CAD build for the part. Positions are in the model's coordinates, mm. Face numbers are marked on the shaded views. A direction names the side the tool comes from. Round coordinates to 2 decimals unless told otherwise and drop trailing zeros. Write each loop counter-clockwise with the first axis right and the second up, starting at its lowest first coordinate (ties: lowest second). Pieces come first, ordered by that corner, then holes. Notation, with made-up numbers: (6.25, -13) - (14.25, -13) arc R14 cw to (14.25, 6) - close; hole circle Ø10 at (-18.5, 67.5). An arc over 180 degrees is marked (long way). Answer in a Markdown table with one row per item.
```python
from build123d import *

# Parameters (mm, degrees)
BOSS_EXTRUDE1_DEPTH = 241.3
FILLET1_R           = 25.4
FILLET2_R           = 12.7
CUT_EXTRUDE1_DEPTH  = 558.8
SKETCH3_W           = 1114.093901139
SKETCH3_H           = 2455.440787086
CUT_EXTRUDE5_DEPTH  = 101.6
SKETCH4_W           = 139.7
SKETCH4_H           = 12.7
CUT_EXTRUDE6_DEPTH  = 401.32
SKETCH9_W           = 863.6
SKETCH9_H           = 101.6
SKETCH9_W_2         = 342.9
SKETCH9_H_2         = 914.4
BOSS_EXTRUDE5_DEPTH = 254
SKETCH10_W          = 76.2
SKETCH10_H          = 76.2
BOSS_EXTRUDE6_DEPTH = 914.4


with BuildPart() as part:
    # Sketch1 → Boss-Extrude1 (new body)
    with BuildSketch(Plane.XY):
        Polygon((977.9, -152.4), (419.1, -152.4), (419.1, -2159), (977.9, -2159), (977.9, -2311.4), (0, -2311.4), (0, 0), (977.9, 0), align=None)
    extrude(amount=BOSS_EXTRUDE1_DEPTH)

    # Fillet1
    fillet1_edges = [part.edges().sort_by_distance(p)[0] for p in [
        (419.1, -152.4, 120.65),
        (419.1, -2159, 120.65),
    ]]
    fillet(fillet1_edges, radius=FILLET1_R)

    # Fillet2
    fillet2_edges = [part.edges().sort_by_distance(p)[0] for p in [
        (977.9, -2235.2, 241.3),
        (0, 0, 120.65),
        (977.9, 0, 120.65),
        (977.9, -152.4, 120.65),
        (977.9, -2159, 120.65),
        (977.9, -2311.4, 120.65),
        (0, -2311.4, 120.65),
        (977.9, -76.2, 241.3),
        (977.9, -76.2, 0),
        (977.9, -2235.2, 0),
    ]]
    fillet(fillet2_edges, radius=FILLET2_R)

    # Sketch2 → Cut-Extrude1 (cut)
    with BuildSketch(Plane(origin=(977.9, 0, 0), x_dir=(0, 0, -1), z_dir=(1, 0, 0))):
        with BuildLine():
            Line((-196.85, -152.4), (-196.85, -114.3))
            ThreePointArc((-196.85, -114.3), (-158.73, -85.205737384), (-120.61, -114.3))
            Line((-120.61, -114.3), (-120.61, -152.4))
            Line((-120.61, -152.4), (-196.85, -152.4))
        make_face()
    cut_extrude1 = extrude(amount=-CUT_EXTRUDE1_DEPTH, mode=Mode.SUBTRACT)

    # Mirror1: Cut-Extrude1 across plane
    add(cut_extrude1.mirror(Plane.ZX.offset(-1155.7)), mode=Mode.SUBTRACT)

    # Sketch3 → Cut-Extrude5 (cut)
    with BuildSketch(Plane(origin=(0, 0, 0), x_dir=(-1, 0, 0), z_dir=(0, 0, -1))):
        with Locations((-472.168855083, -1170.106383975)):
            Rectangle(SKETCH3_W, SKETCH3_H)
    extrude(amount=-CUT_EXTRUDE5_DEPTH, mode=Mode.SUBTRACT)

    # Sketch4 → Cut-Extrude6 (cut)
    with BuildSketch(Plane(origin=(419.1, 0, 0), x_dir=(0, 0, -1), z_dir=(1, 0, 0))):
        with Locations((-171.45, -673.1)):
            Rectangle(SKETCH4_W, SKETCH4_H)
    cut_extrude6 = extrude(amount=-CUT_EXTRUDE6_DEPTH, mode=Mode.SUBTRACT)

    # Mirror2: Cut-Extrude6 across plane
    add(cut_extrude6.mirror(Plane.ZX.offset(-1155.7)), mode=Mode.SUBTRACT)

    # Sketch9 → Boss-Extrude5 (add)
    with BuildSketch(Plane.XY.offset(241.3)):
        with Locations((482.6, -76.2)):
            Rectangle(SKETCH9_W, SKETCH9_H)
        with Locations((209.55, -647.7)):
            Rectangle(SKETCH9_W_2, SKETCH9_H_2)
    boss_extrude5 = extrude(amount=BOSS_EXTRUDE5_DEPTH)

    # Sketch10 → Boss-Extrude6 (add)
    with BuildSketch(Plane.XY.offset(495.3)):
        with Locations((114.3, -76.2)):
            Rectangle(SKETCH10_W, SKETCH10_H)
        with Locations((850.9, -76.2)):
            Rectangle(SKETCH10_W, SKETCH10_H)
        with Locations((190.5, -1028.7)):
            Rectangle(SKETCH10_W, SKETCH10_H)
    boss_extrude6 = extrude(amount=BOSS_EXTRUDE6_DEPTH)

    # Mirror4: Boss-Extrude5, Boss-Extrude6 across plane
    add(boss_extrude5.mirror(Plane.ZX.offset(-1155.7)))
    add(boss_extrude6.mirror(Plane.ZX.offset(-1155.7)))


solid = part.part
```
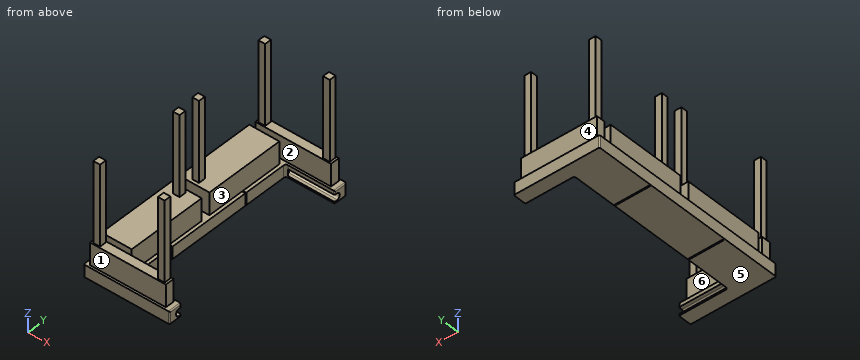
Q1. Saw through at B-B on x = 676. List the corners of the cut face in (y, z).
Computed:
| item | result |
|---|---|
| outline | (-2311.4, 101.6) - (-2159, 101.6) - (-2159, 120.61) - (-2197.1, 120.61) arc R39.52 cw to (-2197.1, 196.85) - (-2159, 196.85) - (-2159, 241.3) - (-2184.4, 241.3) - (-2184.4, 495.3) - (-2286, 495.3) - (-2286, 241.3) - (-2311.4, 241.3) - close; (-152.4, 101.6) - (0, 101.6) - (0, 241.3) - (-25.4, 241.3) - (-25.4, 495.3) - (-127, 495.3) - (-127, 241.3) - (-152.4, 241.3) - (-152.4, 196.85) - (-114.3, 196.85) arc R39.52 cw to (-114.3, 120.61) - (-152.4, 120.61) - close |
Q2. Saw through at D-D on z = 1050.5. List the corners of the cut face in (x, y), then the cut area to 3 significant figures.
Computed:
| item | result |
|---|---|
| outline | (76.2, -2273.3) - (152.4, -2273.3) - (152.4, -2197.1) - (76.2, -2197.1) - close; (76.2, -114.3) - (152.4, -114.3) - (152.4, -38.1) - (76.2, -38.1) - close; (152.4, -1320.8) - (228.6, -1320.8) - (228.6, -1244.6) - (152.4, -1244.6) - close; (152.4, -1066.8) - (228.6, -1066.8) - (228.6, -990.6) - (152.4, -990.6) - close; (812.8, -2273.3) - (889, -2273.3) - (889, -2197.1) - (812.8, -2197.1) - close; (812.8, -114.3) - (889, -114.3) - (889, -38.1) - (812.8, -38.1) - close |
| area | 34,800 mm2 |
Q3. Flat gauge pins, fed straight in: pin 1 (19 mm diameter, centred on x = 799.5, y = -2177.5, fed in from +Z); pin 2 (10 mm diameter, centred on y = -674, z = 201.5, fed in from +X); pin 3 (12 mm diameter, centred on x = 181.5, z = 936.5, fed in from +Y). Where does each tip first touch, or does it go through?
Computed:
| item | result |
|---|---|
| pin 1 | stops at z = 495.3 |
| pin 2 | stops at x = 17.78 |
| pin 3 | stops at y = -990.6 |
Q4. Drill centre lines: line 1 (Y direction, x = 253, z = 167); line 2 (Z direction, x = 809, y = -113.5); line 3 (Y direction, x = 250, z = 402.5). Where is each one in solid material? Low to high.
Computed:
| item | result |
|---|---|
| line 1 | y = -2311.4 to -1644.65, -1631.95 to -679.45, -666.75 to 0 |
| line 2 | z = 101.6 to 120.84, 196.62 to 495.3 |
| line 3 | y = -2286 to -2184.4, -2120.9 to -1206.5, -1104.9 to -190.5, -127 to -25.4 |
Q5. 3-axis set-ups, long thin cutter, end or side, ignore diameter. For the marked faces 1, 2 and 3: which of +Z, -Z, +X, -X, +Y, -Y reach the whole face in a straight line?
Computed:
| item | result |
|---|---|
| face 1 | +Z, +X, -X, -Y |
| face 2 | +Z, +X, -X |
| face 3 | +Z, +X |
Q6. Saw through at C-C on y = -430. List the corners of the cut face in (x, z), then the cut area to 3 significant figures.
Computed:
| item | result |
|---|---|
| outline | (0, 101.6) - (419.1, 101.6) - (419.1, 241.3) - (381, 241.3) - (381, 495.3) - (38.1, 495.3) - (38.1, 241.3) - (0, 241.3) - close |
| area | 146,000 mm2 |
Q7. Pull direction Y, two halves, no side cores. Call the marked faces 4, 5 and 6: released by +Y, released by -Y, zero draft, split by the parting line, or undercut.
Computed:
| item | result |
|---|---|
| face 4 | released by +Y |
| face 5 | zero draft |
| face 6 | undercut |
Q8. Saw through at A-A on z = 328. List the corners of the cut face in (x, y), then the cut area to 3 significant figures.
Computed:
| item | result |
|---|---|
| outline | (38.1, -2120.9) - (381, -2120.9) - (381, -1206.5) - (38.1, -1206.5) - close; (38.1, -1104.9) - (381, -1104.9) - (381, -190.5) - (38.1, -190.5) - close; (50.8, -2286) - (914.4, -2286) - (914.4, -2184.4) - (50.8, -2184.4) - close; (50.8, -127) - (914.4, -127) - (914.4, -25.4) - (50.8, -25.4) - close |
| area | 803,000 mm2 |
